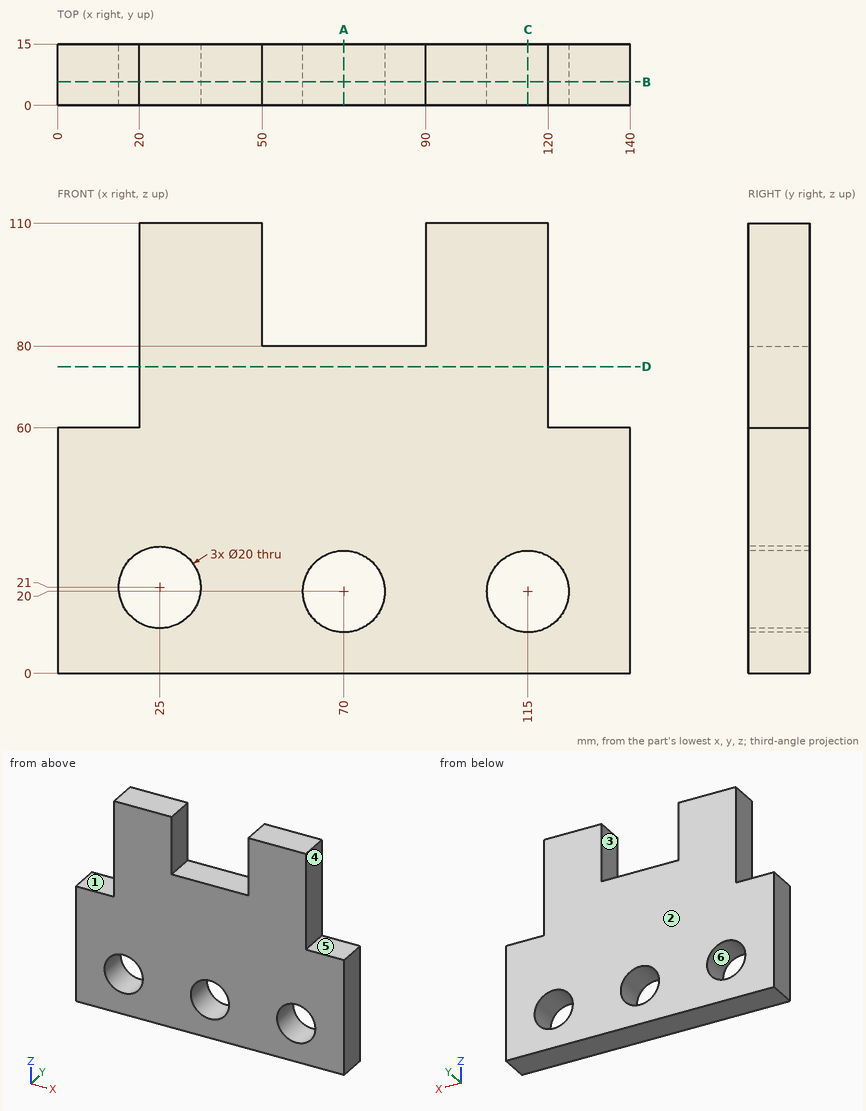
Design review of the part shown in the three views and the two pictorial views. Dimensions are in mm from the part's minimum x, y and z. A direction names the side the tool comes from. Coordinates: 2 decimals unless noted, no trailing zeros. Order: outer loops, then holes, each group sorted by start corner. A loop starts at its lowest first (then second) coordinate and runs counter-clockwise, first axis right, second up. Notation, with made-up numbers: (-4.75, 62) - (33.25, 62) arc R7 ccw to (33.25, 73) - close; hole circle Ø10 at (56.25, 85.25). An arc over 180 degrees is marked (long way). Answer as CSV lines item,"result". Start each with the question number.
1) Draft analysis for pull direction Z (two halves, no side actions). For the marked faces 4, 5 and 6, state which applies: +Z half, -Z half, draft (parallel to the pull), parting line (faces both ways), or undercut.
2) Add section C-C (x = 115). State the section outline as (y, z) points, then the cut area to 3 significant figures.
3) Add section A-A (x = 70). State the section outline as (y, z) points, then the cut area to 3 significant figures.
4) Machinability: for the marked faces 1, 2 and 3, which of the approach directions +Z, -Z, +X, -X, +Y, -Y give a long, thin tool a straight path to every point of the face, cutting with its end or side? Answer none if there is none.
5) Add section B-B (y = 5.75). State the section outline as (x, z) points, then the cut area to 3 significant figures.
6) Insertion check: P1, Ø4.5, axis at y = 10.5, z = 92.5, coming from the -X side; P2, Ø1.5, axis at x = 122, y = 10.5, coming from the +Z side; P3, Ø16, axis at x = 70, z = 20, coming from the +Y side. Each pin has a flat end and moves straight along its axis. Give the tip position at first contact, or say it passes through.
7) To check wall thickness, follow line 1 along Z through (x, y) = (70, 9.5); line 2 along X through (y, z) = (8.5, 99); line 3 along Z through (x, y) = (25, 5.75). State the ranges of each line that lie inside material, in increasing order. Write a range as [from, to].
8) Add section D-D (z = 75). State the section outline as (x, y) points.
Result:
1,face 4,"draft"
1,face 5,"+Z half"
1,face 6,"undercut"
2,outline,"(0, 0) - (15, 0) - (15, 10) - (0, 10) - close; (0, 30) - (15, 30) - (15, 110) - (0, 110) - close"
2,area,"1,350 mm^2"
3,outline,"(0, 0) - (15, 0) - (15, 10) - (0, 10) - close; (0, 30) - (15, 30) - (15, 80) - (0, 80) - close"
3,area,"900 mm^2"
4,face 1,"+Z, -X, +Y, -Y"
4,face 2,"+Z, -Z, +X, -X, +Y"
4,face 3,"+Z, +Y, -Y"
5,outline,"(0, 0) - (140, 0) - (140, 60) - (120, 60) - (120, 110) - (90, 110) - (90, 80) - (50, 80) - (50, 110) - (20, 110) - (20, 60) - (0, 60) - close; hole circle Ø20 at (25, 21); hole circle Ø20 at (70, 20); hole circle Ø20 at (115, 20)"
5,area,"11,300 mm^2"
6,P1,"x = 20"
6,P2,"z = 60"
6,P3,"through"
7,line 1,"[0, 10], [30, 80]"
7,line 2,"[20, 50], [90, 120]"
7,line 3,"[0, 11], [31, 110]"
8,outline,"(20, 0) - (120, 0) - (120, 15) - (20, 15) - close"
